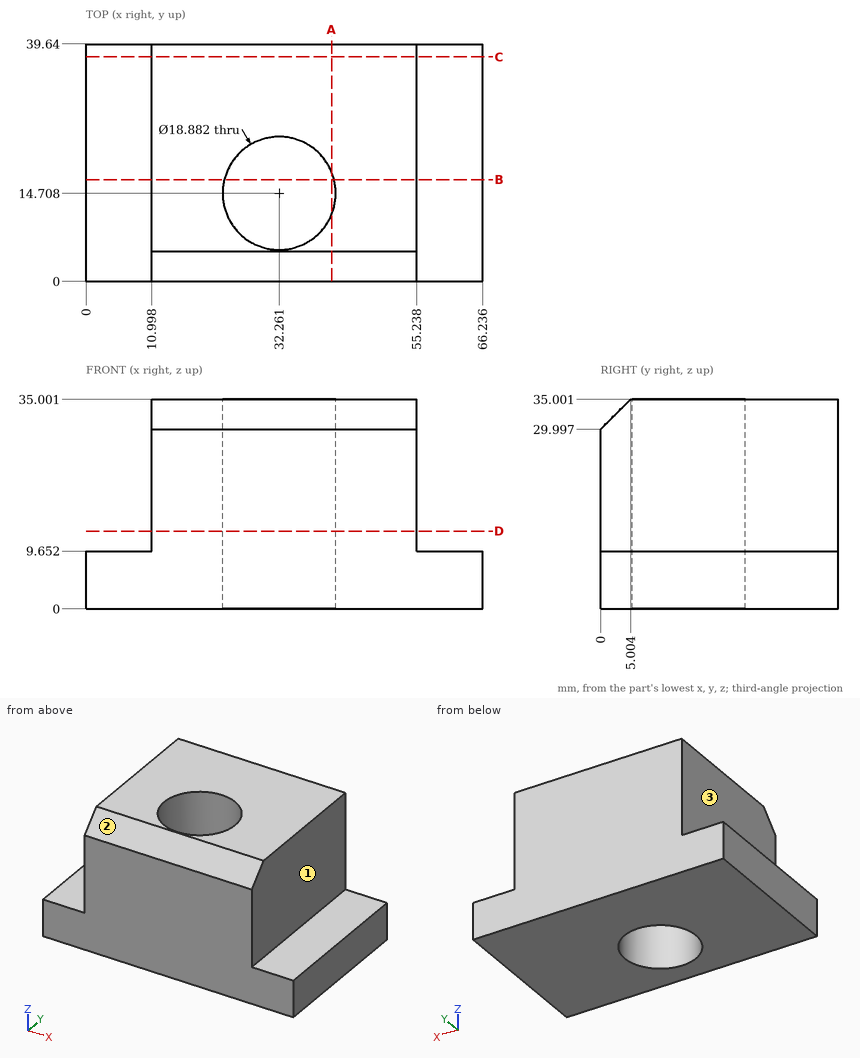
Study the drawing (mm; zero at the part's minimum x, y, z) and answer. A direction names the side the tool comes from. Give positions to 0.01 mm unless a question says otherwise; leave off trailing zeros. Order: outer loops, then holes, each group sorted by start corner. A loop starts at its lowest first (then second) coordinate and runs counter-clockwise, first axis right, second up.
1) Given P1, Ø5, axis at x = 29.5, z = 3.5, coming from the -Y side; P2, Ø15, axis at x = 32.26, y = 14.71, coming from the +Z side; P3, Ø1.5, axis at y = 21, z = 22.5, coming from the -X side; P4, Ø3.5, axis at x = 3, y = 27, coming from the +Z side, each flat-ended and moving along its own axis, determine where each tip first touches the part or whether it passes through.
Reported:
P1: stops at y = 0
P2: passes through
P3: stops at x = 11
P4: stops at z = 9.65
2) Find section C-C on y = 37.5. Write down the section's boundary in (x, z).
Reported:
outline: (0, 0) - (66.24, 0) - (66.24, 9.65) - (55.24, 9.65) - (55.24, 35) - (11, 35) - (11, 9.65) - (0, 9.65) - close
3) For the marked faces 1, 2 and 3, determine the directions among +Z, -Z, +X, -X, +Y, -Y from which every point of the face is accessible in a straight line to the end or side of a thin tool.
Reported:
face 1: +Z, +X, +Y, -Y
face 2: +Z, +X, -X, -Y
face 3: +Z, -X, +Y, -Y
4) Find section D-D on z = 13. Write down the section's boundary in (x, y).
Reported:
outline: (11, 0) - (55.24, 0) - (55.24, 39.64) - (11, 39.64) - close; hole circle Ø18.88 at (32.26, 14.71)
5) Consider line 1 along Z through (x, y) = (56.5, 25.5); line 2 along Y through (x, z) = (38, 16) (1 decimal); line 3 along X through (y, z) = (15, 14) (1 decimal). Determine where each line is inside the solid, lowest interval first.
Reported:
line 1: z = 0 to 9.65
line 2: y = 0 to 7.2, 22.2 to 39.6
line 3: x = 11 to 22.8, 41.7 to 55.2
6) Find section B-B on y = 17. Write down the section's boundary in (x, z).
Reported:
outline: (0, 0) - (23.1, 0) - (23.1, 35) - (11, 35) - (11, 9.65) - (0, 9.65) - close; (41.42, 0) - (66.24, 0) - (66.24, 9.65) - (55.24, 9.65) - (55.24, 35) - (41.42, 35) - close
7) Find section A-A on x = 41. Write down the section's boundary in (y, z), then the cut area to 4 significant figures.
Reported:
outline: (0, 0) - (11.14, 0) - (11.14, 35) - (5, 35) - (0, 30) - close; (18.28, 0) - (39.64, 0) - (39.64, 35) - (18.28, 35) - close
area: 1,125 mm2
